Model file for the job. Use its own axes, mm. Coordinates: 2 decimals unless noted, no trailing zeros. Write each loop counter-clockwise with the first axis right and the second up, starting at its lowest first coordinate (ties: lowest second). Pieces come first, ordered by that corner, then holes. Notation, with made-up numbers: M 12.5,-1 L 69.5,-1 A20 cw 69.5,23 Z; hole C 25,-7 d2. An arc over 180 degrees is marked long. Answer in a Markdown table with one row per item. Add a question column.
```python
from build123d import *

# Parameters (mm, degrees)
SKETCH1_W           = 34.925
SKETCH1_H           = 3.175
BOSS_EXTRUDE1_DEPTH = 3.175
FILLET1_RADIUS      = 1.5875
FILLET1_LENGTH      = 3.175
FILLET2_RADIUS      = 1.5875
FILLET2_LENGTH      = 3.175


with BuildPart() as part:
    # Sketch1 → Boss-Extrude1 (new body)
    with BuildSketch(Plane(origin=(0, 0, 0), x_dir=(0, 0, -1), z_dir=(1, 0, 0))):
        with Locations((17.4625, 1.5875)):
            Rectangle(SKETCH1_W, SKETCH1_H)
    extrude(amount=BOSS_EXTRUDE1_DEPTH)

    # Fillet1: full round fillet: the end face becomes a half cylinder, R = half its width
    fillet1_face = Plane((1.5875, 1.5875, 0), x_dir=(0, 1, 0), z_dir=(0, 0, 1))  # on the end face: x along it, z out of the body
    fillet1_slab = fillet1_face.offset(-FILLET1_RADIUS / 2) * Box(FILLET1_LENGTH, 2 * FILLET1_RADIUS, FILLET1_RADIUS, mode=Mode.PRIVATE)  # the body's end, R deep
    fillet1_round = Plane((1.5875, 1.5875, -1.5875), x_dir=(0, 0, 1), z_dir=(0, 1, 0)) * Cylinder(FILLET1_RADIUS, FILLET1_LENGTH, mode=Mode.PRIVATE)  # its axis R under the face
    add(fillet1_slab - fillet1_round, mode=Mode.SUBTRACT)

    # Fillet2: full round fillet: the end face becomes a half cylinder, R = half its width
    fillet2_face = Plane((1.5875, 1.5875, -34.925), x_dir=(0, -1, 0), z_dir=(0, 0, -1))  # on the end face: x along it, z out of the body
    fillet2_slab = fillet2_face.offset(-FILLET2_RADIUS / 2) * Box(FILLET2_LENGTH, 2 * FILLET2_RADIUS, FILLET2_RADIUS, mode=Mode.PRIVATE)  # the body's end, R deep
    fillet2_round = Plane((1.5875, 1.5875, -33.3375), x_dir=(0, 0, -1), z_dir=(0, -1, 0)) * Cylinder(FILLET2_RADIUS, FILLET2_LENGTH, mode=Mode.PRIVATE)  # its axis R under the face
    add(fillet2_slab - fillet2_round, mode=Mode.SUBTRACT)


solid = part.part
```
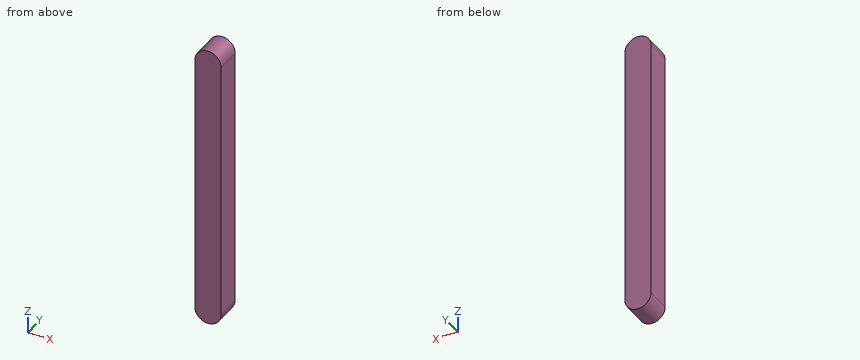
1) Slice it at A-A (y = 1.5). Give the cut face in (x, z) (1 decimal), then the cut area to 3 significant figures.
2) Flat gauge pin, fed straight in: pin 1 Ø1.5 at (x, y) = (2.5, 2) entering from -Z. Where does the tip first touch, or does it go through?
3) Slice it at B-B (x = 0.5). Give the cut face in (y, z) (3 decimals).
4) Drill centre lines: probe 1 along X at (y, z) = (0.4, -1.5); probe 2 along Z at (x, y) = (1.1, 2.9); probe 3 along Z at (x, y) = (2.05, 2.95). Where is each one in solid material? Low to high.
Ans:
| question | item | result |
|---|---|---|
| 1 | outline | M 0,-33.3 A1.6 ccw 3.2,-33.3 L 3.2,-1.6 A1.6 ccw 0,-1.6 Z |
| 1 | area | 109 mm2 |
| 2 | pin 1 | stops at z = -34.92 |
| 3 | outline | M 0,-34.494 L 3.175,-34.494 L 3.175,-0.431 L 0,-0.431 Z |
| 4 | probe 1 | x = 0 to 3.17 |
| 4 | probe 2 | z = -34.85 to -0.08 |
| 4 | probe 3 | z = -34.86 to -0.07 |
